Geometry check sheet. Reference: drawing and pictorial views, mm from the part's lowest x, y, z. A direction names the side the tool comes from. Coordinates: 2 decimals unless noted, no trailing zeros. Loops run counter-clockwise (first coordinate to the right, second up) from the corner with the lowest first, then second, coordinate; pieces in that order, holes last. Notation, with made-up numbers: (-16, 68) - (-10, 68) arc R13 ccw to (-10, 88) - close; hole circle Ø1 at (51.5, 57). An arc over 180 degrees is marked (long way). One line per item, written item: value.
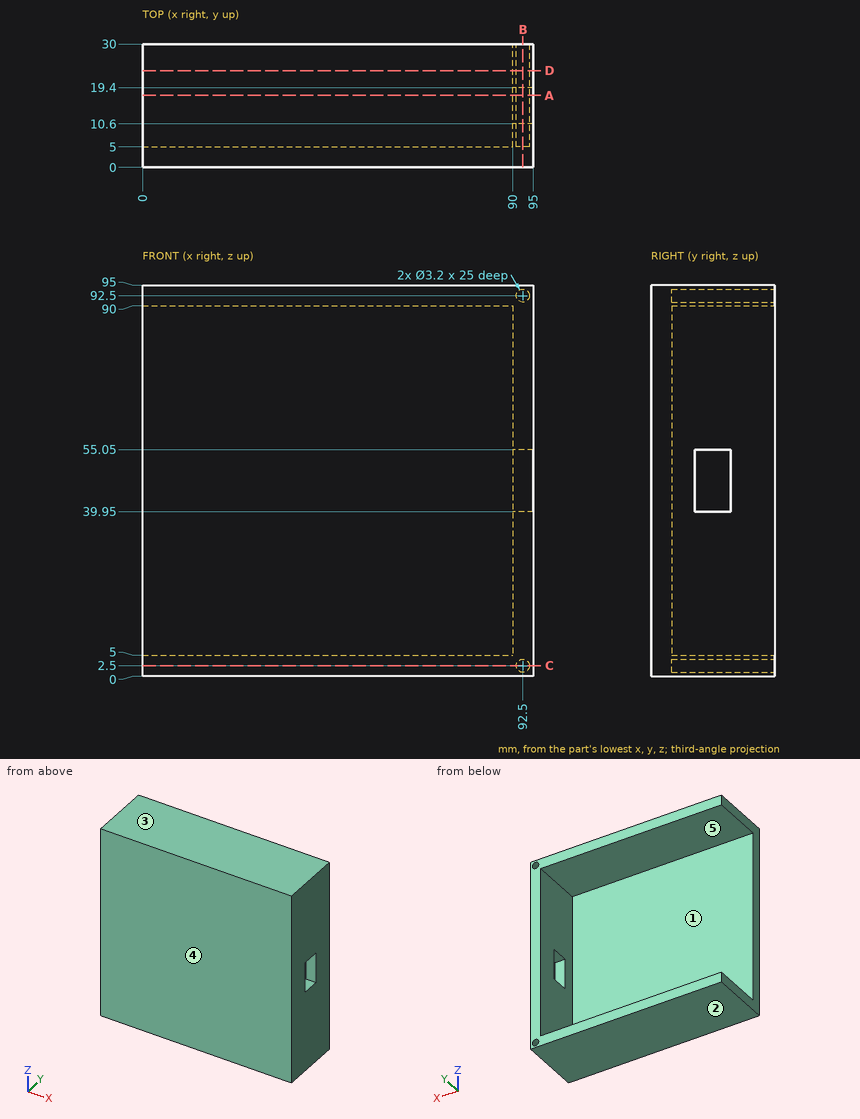
(1) Release check for a two-part mould opening along Z. For the marked faces 3, 4 and 5 record: pulls with the +Z half, pulls with the -Z half, needs draft (parallel to the pull), parting line crosses it, or undercut.
Reply:
face 3: pulls with the +Z half
face 4: needs draft
face 5: undercut
(2) Access from +Z, -Z, +X, -X, +Y, -Y to the whole of each face (thin tool, end or side, straight path). Record for the marked faces 1 and 2.
Reply:
face 1: -X, +Y
face 2: -Z, +X, -X, +Y, -Y
(3) Go/stop test with flat-tipped pins: pin 1 Ø10 at (x, z) = (34.5, 24.5) entering from +Y; pin 2 Ø10 at (y, z) = (22, 31) entering from -X. Record where each tip stops, or that it passes through.
Reply:
pin 1: y = 5
pin 2: x = 90
(4) Cross-section at C-C on z = 2.5. Record the cut outline in (x, y), and give its area (3 significant figures).
Reply:
outline: (0, 0) - (95, 0) - (95, 30) - (94.1, 30) - (94.1, 5) - (90.9, 5) - (90.9, 30) - (0, 30) - close
area: 2,770 mm2
(5) Material ranges on probe 1 along Z at (x, y) = (92.5, 22); probe 2 along Z at (x, y) = (92.5, 12.75); probe 3 along X at (y, z) = (22.75, 2.5), recorded low to high. Write a range as from..to.
Reply:
probe 1: 0..0.9, 4.1..90.9, 94.1..95
probe 2: 0..0.9, 4.1..39.95, 55.05..90.9, 94.1..95
probe 3: 0..90.9, 94.1..95
(6) Cross-section at A-A on y = 17.5. Record the cut outline in (x, z), and give its area (3 significant figures).
Reply:
outline: (0, 0) - (95, 0) - (95, 39.95) - (90, 39.95) - (90, 5) - (0, 5) - close; (0, 90) - (90, 90) - (90, 55.05) - (95, 55.05) - (95, 95) - (0, 95) - close; hole circle Ø3.2 at (92.5, 2.5); hole circle Ø3.2 at (92.5, 92.5)
area: 1,280 mm2
(7) Cross-section at D-D on y = 23.5. Record the cut outline in (x, z), and give its area (3 significant figures).
Reply:
outline: (0, 0) - (95, 0) - (95, 95) - (0, 95) - (0, 90) - (90, 90) - (90, 5) - (0, 5) - close; hole circle Ø3.2 at (92.5, 2.5); hole circle Ø3.2 at (92.5, 92.5)
area: 1,360 mm2
(8) Cross-section at B-B on x = 92.5. Record the cut outline in (y, z).
Reply:
outline: (0, 0) - (30, 0) - (30, 0.9) - (5, 0.9) - (5, 4.1) - (30, 4.1) - (30, 90.9) - (5, 90.9) - (5, 94.1) - (30, 94.1) - (30, 95) - (0, 95) - close; hole (10.6, 39.95) - (19.4, 39.95) - (19.4, 55.05) - (10.6, 55.05) - close
